Job drawing, mm, ordinate dimensions from the low corner. One solid piece. A direction names the side the tool comes from. Round coordinates to 2 decimals unless told otherwise and drop trailing zeros. Loops run counter-clockwise (first coordinate to the right, second up) from the corner with the lowest first, then second, coordinate; pieces in that order, holes last.
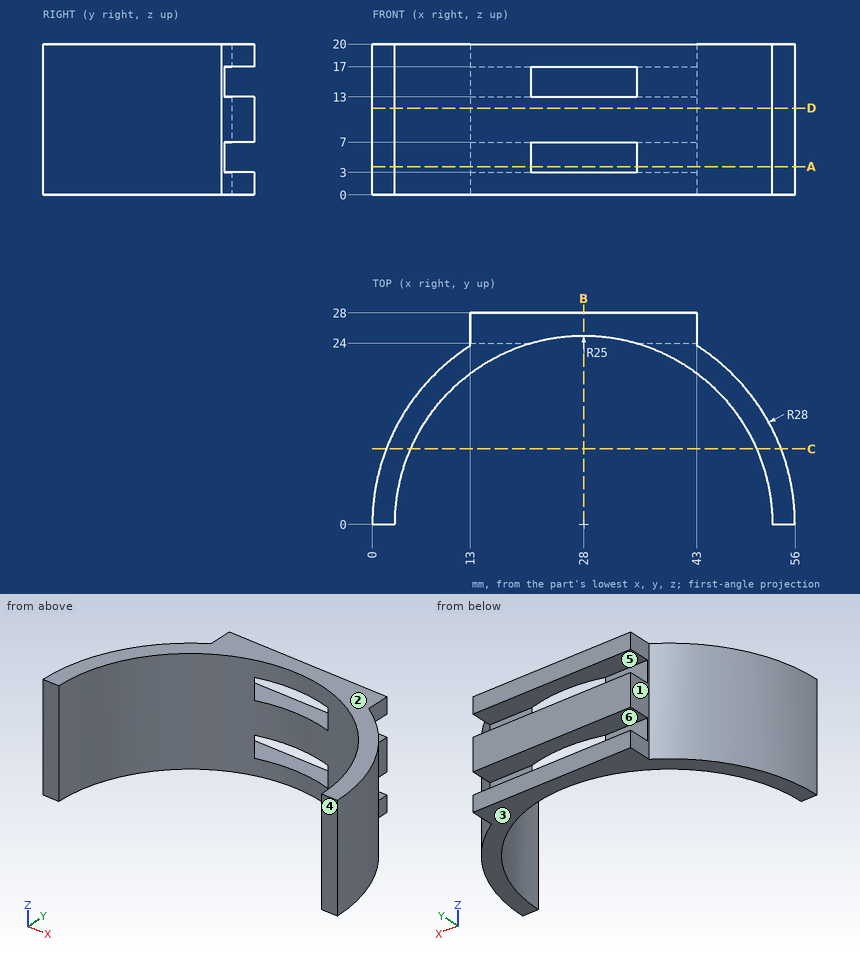
(1) Slice it at A-A on z = 3.75. List the corners of the cut face in (x, y).
Responses:
outline: (0, 0) - (3, 0) arc R25 cw to (21, 24) - (13, 24) - (13, 23.64) arc R28 ccw to start; (35, 24) arc R25 cw to (53, 0) - (56, 0) arc R28 ccw to (43, 23.64) - (43, 24) - close
(2) Which spindle directions (+Z, -Z, +X, -X, +Y, -Y) get a long thin tool onto all of the face, cutting with end or side? Do the marked faces 1 and 2. Say none if no direction does.
Responses:
face 1: +Z, -Z, -X, +Y
face 2: +Z, +X, -X, +Y, -Y
(3) Pin check, flat tips, straight feed: P1, Ø1, axis at x = 19, z = 15.5, coming from the +Y side; P2, Ø12, axis at x = 17, z = 5, coming from the -Y side; P3, Ø4.5, axis at x = 18.5, z = 5.5, coming from the +Y side; P4, Ø2, axis at y = 10.5, z = 5.5, coming from the +X side. Stop position of each tip, or through.
Responses:
P1: stops at y = 24
P2: stops at y = 18.33
P3: stops at y = 28
P4: stops at x = 54.34
(4) Slice it at B-B on x = 28. List the corners of the cut face in (y, z), plus the area to 3 significant figures.
Responses:
outline: (25, 0) - (28, 0) - (28, 3) - (25, 3) - close; (25, 7) - (28, 7) - (28, 13) - (25, 13) - close; (25, 17) - (28, 17) - (28, 20) - (25, 20) - close
area: 36.0 mm2
(5) Pull direction Z, two halves, no side cores. Call the marked faces 3, 4, 5 and 6: +Z half, -Z half, draft (parallel to the pull), parting line (faces both ways), or undercut.
Responses:
face 3: -Z half
face 4: draft
face 5: undercut
face 6: undercut
(6) Slice it at D-D on z = 11.5. List the corners of the cut face in (x, y).
Responses:
outline: (0, 0) - (3, 0) arc R25 cw to (53, 0) - (56, 0) arc R28 ccw to (43, 23.64) - (43, 28) - (13, 28) - (13, 23.64) arc R28 ccw to start
(7) Slice it at C-C on y = 10. List the corners of the cut face in (x, z), plus the area to 3 significant figures.
Responses:
outline: (1.85, 0) - (5.09, 0) - (5.09, 20) - (1.85, 20) - close; (50.91, 0) - (54.15, 0) - (54.15, 20) - (50.91, 20) - close
area: 130 mm2
(8) Probe line 1 (X direction, y = 5.25, z = 1); line 2 (X direction, y = 23, z = 8.5); line 3 (Y direction, x = 11.5, z = 3.25). List the from-to ranges inside material, lowest first.
Responses:
line 1: x = 0.5 to 3.56, 52.44 to 55.5
line 2: x = 12.03 to 18.2, 37.8 to 43.97
line 3: y = 18.78 to 22.62
